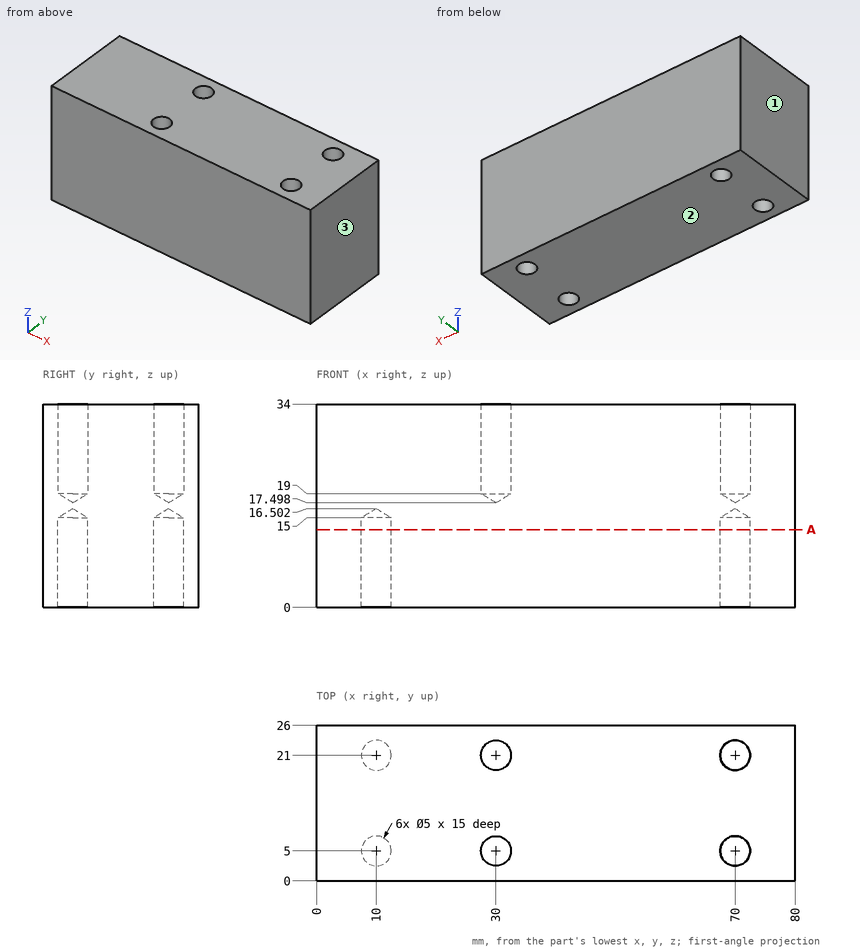
Verification items for this drawing (mm, ordinates from the low corner). Coordinates: 2 decimals unless noted, no trailing zeros. Order: outer loops, then holes, each group sorted by start corner. A loop starts at its lowest first (then second) coordinate and runs counter-clockwise, first axis right, second up. Notation, with made-up numbers: (-27.5, 72) - (31.5, 72) arc R18 ccw to (31.5, 102) - close; hole circle Ø9 at (-27.75, -39.5). An arc over 180 degrees is marked (long way). Answer in a Markdown table with one row per item. Add a question column.
1. Section check A-A (z = 13). Enter the section's corners in (x, y).
2. Draft check along X on the marked faces 1, 2 and 3. Enter one of: +X half, -X half, draft (parallel to the pull), parting line (faces both ways), or undercut.
3. Gauge pin test, flat ends, axial feed: pin 1 Ø4 at (x, y) = (70, 21) entering from -Z; pin 2 Ø4.5 at (x, y) = (70, 5) entering from -Z; pin 3 Ø4 at (x, y) = (70, 5) entering from +Z. Record the tip position at first contact, or that the pin passes through.
4. Material ranges on L1, parallel to Y at x = 10, z = 6; L2, parallel to X at y = 21, z = 28; L3, parallel to X at y = 4, z = 7, recorded low to high. Write a range as [from, to].
Data:
| question | item | result |
|---|---|---|
| 1 | outline | (0, 0) - (80, 0) - (80, 26) - (0, 26) - close; hole circle Ø5 at (10, 5); hole circle Ø5 at (10, 21); hole circle Ø5 at (70, 5); hole circle Ø5 at (70, 21) |
| 2 | face 1 | -X half |
| 2 | face 2 | draft |
| 2 | face 3 | +X half |
| 3 | pin 1 | stops at z = 15.3 |
| 3 | pin 2 | stops at z = 15.15 |
| 3 | pin 3 | stops at z = 18.7 |
| 4 | L1 | y = [0, 2.5], [7.5, 18.5], [23.5, 26] |
| 4 | L2 | x = [0, 27.5], [32.5, 67.5], [72.5, 80] |
| 4 | L3 | x = [0, 7.71], [12.29, 67.71], [72.29, 80] |
